from build123d import *

# Parameters (mm, degrees)
SKETCH_1_R               = 27.5
SKETCH_1_R_2             = 10
EXTRUDE_1_DEPTH          = 10
SKETCH_2_R               = 27.5
EXTRUDE_2_DEPTH          = 10
SKETCH_3_W               = 8
SKETCH_3_H               = 2.5
CUT_EXTRUDE_2_DEPTH      = 108
PATTERN_CIRCULAR_2_COUNT = 6


with BuildPart() as part:
    # Sketch 1 → Extrude 1 (new body)
    with BuildSketch(Plane(origin=(0, 0, 0), x_dir=(1, 0, 0), z_dir=(0, 1, 0))):
        with BuildLine():
            ThreePointArc((36.626693786, -26.14355183), (45, 0), (36.626693786, 26.14355183))
            ThreePointArc((36.626693786, 26.14355183), (35.489388485, 31.722157226), (38.87340923, 36.300661906))
            ThreePointArc((38.87340923, 36.300661906), (42.889809267, 64.52547333), (14.571428571, 61.232941793))
            ThreePointArc((14.571428571, 61.232941793), (0, 52.989280604), (-14.571428571, 61.232941793))
            ThreePointArc((-14.571428571, 61.232941793), (-42.889809267, 64.52547333), (-38.87340923, 36.300661906))
            ThreePointArc((-38.87340923, 36.300661906), (-35.489388485, 31.722157226), (-36.626693786, 26.14355183))
            ThreePointArc((-36.626693786, 26.14355183), (-45, 0), (-36.626693786, -26.14355183))
            ThreePointArc((-36.626693786, -26.14355183), (-35.489388485, -31.722157226), (-38.87340923, -36.300661906))
            ThreePointArc((-38.87340923, -36.300661906), (-42.889809267, -64.52547333), (-14.571428571, -61.232941793))
            ThreePointArc((-14.571428571, -61.232941793), (0, -52.989280604), (14.571428571, -61.232941793))
            ThreePointArc((14.571428571, -61.232941793), (42.889809267, -64.52547333), (38.87340923, -36.300661906))
            ThreePointArc((38.87340923, -36.300661906), (35.489388485, -31.722157226), (36.626693786, -26.14355183))
        make_face()
        with Locations(Location((0, 0, 0), (0, 0, 270))):
            Circle(SKETCH_1_R, mode=Mode.SUBTRACT)
        with Locations(Location((30, -51.961524227, 0), (0, 0, 270))):
            Circle(SKETCH_1_R_2, mode=Mode.SUBTRACT)
        with Locations(Location((-30, -51.961524227, 0), (0, 0, 90))):
            Circle(SKETCH_1_R_2, mode=Mode.SUBTRACT)
        with Locations(Location((-30, 51.961524227, 0), (0, 0, 270))):
            Circle(SKETCH_1_R_2, mode=Mode.SUBTRACT)
        with Locations(Location((30, 51.961524227, 0), (0, 0, 90))):
            Circle(SKETCH_1_R_2, mode=Mode.SUBTRACT)
    extrude(amount=EXTRUDE_1_DEPTH)

    # Sketch 2 → Extrude 2 (add)
    with BuildSketch(Plane(origin=(0, 10, 0), x_dir=(1, 0, 0), z_dir=(0, 1, 0))):
        with BuildLine():
            ThreePointArc((36.626693786, 26.14355183), (0, 45), (-36.626693786, 26.14355183))
            ThreePointArc((-36.626693786, 26.14355183), (-45, 0), (-36.626693786, -26.14355183))
            ThreePointArc((-36.626693786, -26.14355183), (0, -45), (36.626693786, -26.14355183))
            ThreePointArc((36.626693786, -26.14355183), (42.855578519, -13.725865722), (45, 0))
            ThreePointArc((45, 0), (42.855578519, 13.725865722), (36.626693786, 26.14355183))
        make_face()
        with Locations(Location((0, 0, 0), (0, 0, 270))):
            Circle(SKETCH_2_R, mode=Mode.SUBTRACT)
    extrude(amount=EXTRUDE_2_DEPTH)

    # Sketch 3 → Cut-Extrude 2 (cut)
    with BuildSketch(Plane(origin=(0, 0, 0), x_dir=(0, 0, -1), z_dir=(1, 0, 0))):
        with Locations((0, 18.75)):
            Rectangle(SKETCH_3_W, SKETCH_3_H)
    cut_extrude_2 = extrude(amount=-CUT_EXTRUDE_2_DEPTH, mode=Mode.SUBTRACT)

    # Pattern Circular 2: Cut-Extrude 2 ×6 about axis
    pattern_circular_2_axis = Axis((0, 0, 0), (0, 1, 0))
    for i in range(1, PATTERN_CIRCULAR_2_COUNT):
        add(cut_extrude_2.rotate(pattern_circular_2_axis, i * 360 / PATTERN_CIRCULAR_2_COUNT), mode=Mode.SUBTRACT)


solid = part.part
Build history of the part. All positions in model axes, mm. A direction names the side the tool comes from. Coordinates: 2 decimals unless noted, no trailing zeros. Order: outer loops, then holes, each group sorted by start corner. A loop starts at its lowest first (then second) coordinate and runs counter-clockwise, first axis right, second up. Notation, with made-up numbers: (-16.5, -19) - (35.5, -19) arc R15 ccw to (35.5, -7) - close; hole circle Ø7 at (30, -24.75). An arc over 180 degrees is marked (long way). Write each question's results on one line, items separated by ' | '. Start each with the question number.
Item 1: Band-saw the part on C-C on x = -30. Write the cut outline in (y, z).
Item 2: Band-saw the part on A-A on x = 0. Write the cut outline in (y, z).
Item 3: Tool access for faces 1 (the face through (-21.41, 18.73, 29.08)), 2 (the face through (-1, 10, -48)), 3 (the face through (36, 17.5, 0)): list every direction of +Z, -Z, +X, -X, +Y, -Y with a clear straight run to the whole face (end or side of a thin tool).
Item 4: Wall check: probe 1 along X at (y, z) = (5.5, 47); probe 2 along X at (y, z) = (7.5, -45); probe 3 along X at (y, z) = (5.25, 0). Give the ranges that are in metal, low to high. Write a range as [from, to].
Item 5: Band-saw the part on B-B on y = 4.75. Write the cut outline in (x, z).
Item 6: Mould opens along X. For faces 4 (the face through (43.2, 4.9, -64.2)), 5 (the face through (-35.508, 4.93, -31.802)), 6 (the face through (-31, 20, 17)) say: released by +X, released by -X, zero draft, split by the parting line, or undercut.
Item 7: Flat gauge pins, fed straight in: pin 1 (6 mm diameter, centred on x = -32, y = 8.5, fed in from +Z); pin 2 (4 mm diameter, centred on x = 29.5, y = 17, fed in from +Z); pin 3 (0.8 mm diameter, centred on x = -35.5, y = 19, fed in from -Z); pin 4 (1.2 mm diameter, centred on x = 34, y = 19, fed in from +Z). Where does each tip first touch, or does it go through?
Numbers:
1) outline: (0, -69.96) - (10, -69.96) - (10, -61.96) - (0, -61.96) - close; (0, -41.96) - (10, -41.96) - (10, -33.54) - (20, -33.54) - (20, -4) - (17.5, -4) - (17.5, 4) - (20, 4) - (20, 33.54) - (10, 33.54) - (10, 41.96) - (0, 41.96) - close; (0, 61.96) - (10, 61.96) - (10, 69.96) - (0, 69.96) - close
2) outline: (0, -52.99) - (10, -52.99) - (10, -45) - (20, -45) - (20, -27.5) - (0, -27.5) - close; (0, 27.5) - (20, 27.5) - (20, 45) - (10, 45) - (10, 52.99) - (0, 52.99) - close
3) face 1: +Y | face 2: -Z, +Y | face 3: +X, -X, +Y
4) probe 1: [-47.3, -38.68], [-21.32, 21.32], [38.68, 47.3] | probe 2: [-46.6, -37.18], [-22.82, 22.82], [37.18, 46.6] | probe 3: [-45, -27.5], [27.5, 45]
5) outline: (-38.87, -36.3) arc R18 ccw (long way) to (-14.57, -61.23) arc R17 cw to (14.57, -61.23) arc R18 ccw (long way) to (38.87, -36.3) arc R7 cw to (36.63, -26.14) arc R45 ccw to (36.63, 26.14) arc R7 cw to (38.87, 36.3) arc R18 ccw (long way) to (14.57, 61.23) arc R17 cw to (-14.57, 61.23) arc R18 ccw (long way) to (-38.87, 36.3) arc R7 cw to (-36.63, 26.14) arc R45 ccw to (-36.63, -26.14) arc R7 cw to start; hole circle Ø20 at (-30, -51.96); hole circle Ø20 at (-30, 51.96); hole circle Ø55 at (0, 0); hole circle Ø20 at (30, -51.96); hole circle Ø20 at (30, 51.96)
6) face 4: undercut | face 5: released by -X | face 6: zero draft
7) pin 1: z = 69.96 | pin 2: z = 35.62 | pin 3: z = -28.16 | pin 4: z = 30.16
